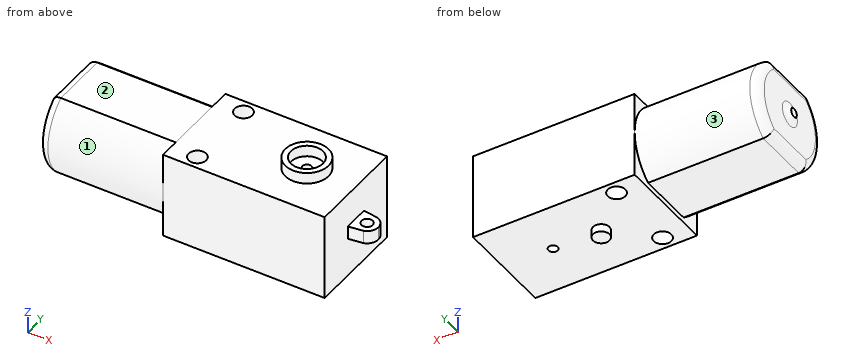
```python
from build123d import *

# Parameters (mm, degrees)
SKETCH1_W           = 18.3388
SKETCH1_H           = 22.3266
BOSS_EXTRUDE1_DEPTH = 36.4236
BOSS_EXTRUDE2_DEPTH = 27.94
SKETCH3_R           = 1.0033
BOSS_EXTRUDE3_DEPTH = 0.9398
SKETCH4_W           = 2.9718
SKETCH4_H           = 5.7912
BOSS_EXTRUDE4_DEPTH = 5.08
SKETCH5_R           = 1.27
CUT_EXTRUDE3_DEPTH  = 2.9718
SKETCH7_R           = 4.8768
SKETCH7_R_2         = 3.6195
BOSS_EXTRUDE5_DEPTH = 2.54
SKETCH9_W           = 36.4236
SKETCH9_H           = 22.3266
BOSS_EXTRUDE6_DEPTH = 1.1938
SKETCH8_R           = 1.0414
SKETCH8_R_2         = 1.9812
CUT_EXTRUDE4_DEPTH  = 19.5326
SKETCH10_R          = 1.8542
BOSS_EXTRUDE7_DEPTH = 1.7526
SKETCH11_W          = 30.653846682
SKETCH11_H          = 27.216421179
CUT_EXTRUDE5_DEPTH  = 0.1
FILLET1_R           = 2


with BuildPart() as part:
    # Sketch1 → Boss-Extrude1 (new body)
    with BuildSketch(Plane(origin=(0, 0, 0), x_dir=(0, 0, -1), z_dir=(1, 0, 0))):
        Rectangle(SKETCH1_W, SKETCH1_H)
    extrude(amount=BOSS_EXTRUDE1_DEPTH)

    # Sketch2 → Boss-Extrude2 (add)
    with BuildSketch(Plane.ZY):
        with BuildLine():
            Line((-9.1694, -6.367210577), (-9.1694, 6.367210577))
            ThreePointArc((-9.1694, 6.367210577), (0, 11.1633), (9.1694, 6.367210577))
            Line((9.1694, 6.367210577), (9.1694, -6.367210577))
            ThreePointArc((9.1694, -6.367210577), (0, -11.1633), (-9.1694, -6.367210577))
        make_face()
    extrude(amount=BOSS_EXTRUDE2_DEPTH)

    # Sketch3 → Boss-Extrude3 (add)
    with BuildSketch(Plane.ZY.offset(27.94)):
        Circle(SKETCH3_R)
    extrude(amount=BOSS_EXTRUDE3_DEPTH)

    # Sketch4 → Boss-Extrude4 (add)
    with BuildSketch(Plane(origin=(36.4236, 0, 0), x_dir=(0, 0, -1), z_dir=(1, 0, 0))):
        Rectangle(SKETCH4_W, SKETCH4_H)
    extrude(amount=BOSS_EXTRUDE4_DEPTH)

    # Sketch5 → Cut-Extrude3 (cut)
    with BuildSketch(Plane.XY.offset(1.4859)):
        with BuildLine():
            Line((36.4236, 2.8956), (39.661128443, 2.442346018))
            ThreePointArc((39.661128443, 2.442346018), (40.991323146, 1.529685864), (41.5036, -2.8e-08))
            Line((41.5036, -2.8e-08), (41.5036, 2.8956))
            Line((41.5036, 2.8956), (36.4236, 2.8956))
        make_face()
        with BuildLine():
            Line((41.5036, -2.8956), (41.5036, -2.8e-08))
            ThreePointArc((41.5036, -2.8e-08), (40.991323129, -1.529685887), (39.661128443, -2.442346018))
            Line((39.661128443, -2.442346018), (36.4236, -2.8956))
            Line((36.4236, -2.8956), (41.5036, -2.8956))
        make_face()
        with Locations((38.9636, 0)):
            Circle(SKETCH5_R)
    extrude(amount=-CUT_EXTRUDE3_DEPTH, mode=Mode.SUBTRACT)

    # Sketch7 → Boss-Extrude5 (add)
    with BuildSketch(Plane.XY.offset(9.1694)):
        with Locations(Location((25.4, 0, 0), (0, 0, 180))):
            Circle(SKETCH7_R)
        with Locations((25.4, 0)):
            Circle(SKETCH7_R_2, mode=Mode.SUBTRACT)
    extrude(amount=BOSS_EXTRUDE5_DEPTH)

    # Sketch9 → Boss-Extrude6 (add)
    with BuildSketch(Plane(origin=(0, 0, -9.1694), x_dir=(-1, 0, 0), z_dir=(0, 0, -1))):
        with Locations((-18.2118, 0)):
            Rectangle(SKETCH9_W, SKETCH9_H)
    extrude(amount=BOSS_EXTRUDE6_DEPTH)

    # Sketch8 → Cut-Extrude4 (cut)
    with BuildSketch(Plane.XY.offset(9.1694)):
        with Locations((25.4, 0)):
            Circle(SKETCH8_R)
        with Locations((5.9182, 8.2423)):
            Circle(SKETCH8_R_2)
        with Locations((5.9182, -8.2423)):
            Circle(SKETCH8_R_2)
    extrude(amount=-CUT_EXTRUDE4_DEPTH, mode=Mode.SUBTRACT)

    # Sketch10 → Boss-Extrude7 (add)
    with BuildSketch(Plane(origin=(0, 0, -10.3632), x_dir=(-1, 0, 0), z_dir=(0, 0, -1))):
        with Locations((-14.5542, 0)):
            Circle(SKETCH10_R)
    extrude(amount=BOSS_EXTRUDE7_DEPTH)

    # Sketch11 → Cut-Extrude5 (cut)
    with BuildSketch(Plane.XY.offset(9.1694)):
        with Locations((-15.326923341, 2.44491059)):
            Rectangle(SKETCH11_W, SKETCH11_H)
    extrude(amount=-CUT_EXTRUDE5_DEPTH, mode=Mode.SUBTRACT)

    # Fillet1
    # the kernel refuses this fillet: 2 mm, written as the material it adds along each edge
    with BuildSketch(Plane(origin=(-27.94, 0, 0), x_dir=(0, 0, 1), z_dir=(0, -1, 0))) as fillet1_piece_1:
        with BuildLine():
            CenterArc((2.699170266, 2), FILLET1_R, 212.012211673, 57.987788327)
            Line((1.0033, 0.9398), (1.0033, 0))
            Line((1.0033, 0), (2.699170266, 0))
        make_face()
    revolve(axis=Axis((-27.94, 0, 0), (-1, 0, 0)))
    # the kernel refuses this fillet: 2 mm, written as the material it takes off along each edge
    with BuildSketch(Plane(origin=(-27.94, -11.367210577, -9.1694), x_dir=(1, 0, 0), z_dir=(0, 1, 0))) as fillet1_2_piece_1:
        with BuildLine():
            CenterArc((FILLET1_R, -FILLET1_R), FILLET1_R, 90, 90)
            Line((0, -FILLET1_R), (0, 0))
            Line((0, 0), (FILLET1_R, 0))
        make_face()
    extrude(amount=22.734421154, mode=Mode.SUBTRACT)
    with BuildSketch(Plane(origin=(-27.94, 0, 0), x_dir=(0, 0.15812676738734943, -0.9874188196685473), z_dir=(0, -0.9874188196685473, -0.15812676738734943))) as fillet1_2_piece_2:
        with BuildLine():
            CenterArc((11.1633 - FILLET1_R, FILLET1_R), FILLET1_R, 270, 90)
            Line((11.1633 - FILLET1_R, 0), (11.1633, 0))
            Line((11.1633, 0), (11.1633, FILLET1_R))
        make_face()
    revolve(axis=Axis((-27.94, 0, 0), (1, 0, 0)), revolution_arc=178.888182092, mode=Mode.SUBTRACT)
    with BuildSketch(Plane(origin=(-27.94, -11.508859388, 9.0694), x_dir=(1, 0, 0), z_dir=(0, 1, 0))) as fillet1_2_piece_3:
        with BuildLine():
            CenterArc((FILLET1_R, FILLET1_R), FILLET1_R, 180, 90)
            Line((0, FILLET1_R), (0, 0))
            Line((0, 0), (FILLET1_R, 0))
        make_face()
    extrude(amount=23.017718776, mode=Mode.SUBTRACT)
    with BuildSketch(Plane(origin=(-27.94, 0, 0), x_dir=(0, 0.1389374526808322, 0.9903011583566695), z_dir=(0, 0.9903011583566695, -0.1389374526808322))) as fillet1_2_piece_4:
        with BuildLine():
            CenterArc((11.1633 - FILLET1_R, FILLET1_R), FILLET1_R, 270, 90)
            Line((11.1633 - FILLET1_R, 0), (11.1633, 0))
            Line((11.1633, 0), (11.1633, FILLET1_R))
        make_face()
    revolve(axis=Axis((-27.94, 0, 0), (1, 0, 0)), revolution_arc=178.888182092, mode=Mode.SUBTRACT)


solid = part.part
```
For this review, take the finished solid that the model builds, in its own axes (mm). Face numbers are marked on the shaded views. A direction names the side the tool comes from. Round coordinates to 2 decimals unless told otherwise and drop trailing zeros. Write each loop counter-clockwise with the first axis right and the second up, starting at its lowest first coordinate (ties: lowest second). Pieces come first, ordered by that corner, then holes.
1) Take a section at C-C on x = -23.5. Give the boundary of the cut face in (y, z), then the cut area to 3 significant figures.
Answer below:
outline: (-6.51, 9.07) arc R11.16 ccw to (-6.37, -9.17) - (6.37, -9.17) arc R11.16 ccw to (6.51, 9.07) - close
area: 356 mm2
2) Machinability: for the marked faces 1, 2 and 3, which of the approach directions +Z, -Z, +X, -X, +Y, -Y give a long, thin tool a straight path to every point of the face, cutting with its end or side? Answer none if there is none.
Answer below:
face 1: -X, -Y
face 2: +Z, -X, +Y, -Y
face 3: -X, +Y
3) Take a section at B-B on x = 6. Give the boundary of the cut face in (y, z), then the cut area to 3 significant figures.
Answer below:
outline: (-11.16, -10.36) - (-10.22, -10.36) - (-10.22, 9.17) - (-11.16, 9.17) - close; (-6.26, -10.36) - (6.26, -10.36) - (6.26, 9.17) - (-6.26, 9.17) - close; (10.22, -10.36) - (11.16, -10.36) - (11.16, 9.17) - (10.22, 9.17) - close
area: 281 mm2
4) Insertion check: pin 1 Ø3 at (x, y) = (-2, -7) entering from +Z; pin 2 Ø6 at (y, z) = (-8, 6.5) entering from +X; pin 3 Ø6.5 at (x, y) = (25, 2) entering from -Z; pin 4 Ø1.5 at (x, y) = (6, -9) entering from -Z. Each pin has a flat end and moves straight along its axis. Give the tip position at first contact, or say it passes through.
Answer below:
pin 1: stops at z = 9.07
pin 2: stops at x = 36.42
pin 3: stops at z = -10.36
pin 4: passes through
5) Take a section at A-A on x = 25.4. Give the boundary of the cut face in (y, z).
Answer below:
outline: (-11.16, -10.36) - (-1.04, -10.36) - (-1.04, 9.17) - (-3.62, 9.17) - (-3.62, 11.71) - (-4.88, 11.71) - (-4.88, 9.17) - (-11.16, 9.17) - close; (1.04, -10.36) - (11.16, -10.36) - (11.16, 9.17) - (4.88, 9.17) - (4.88, 11.71) - (3.62, 11.71) - (3.62, 9.17) - (1.04, 9.17) - close
6) For line 1 along Y through (x, z) = (25.4, 9.7); line 2 along Y through (x, z) = (6, -1); line 3 along Y through (x, z) = (5, 2), list the stretches that pass through material, from the lowest coordinate up.
Answer below:
line 1: y = -4.88 to -3.62, 3.62 to 4.88
line 2: y = -11.16 to -10.22, -6.26 to 6.26, 10.22 to 11.16
line 3: y = -11.16 to -10, -6.49 to 6.49, 10 to 11.16
